Answer from the drawing. Dimensions are ordinates in mm from the lowest x, y and z of the part. Coordinates: 2 decimals unless noted, no trailing zeros. Write each loop counter-clockwise with the first axis right and the second up, starting at its lowest first coordinate (ties: lowest second). Pieces come first, ordered by that corner, then holes. Notation, with made-up numbers: (5, -7) -> (50, -7) arc R18 ccw to (50, 11) -> close; hole circle Ø4 at (60, 56). An arc over 180 degrees is marked (long way). Use CSV: the item, a comma, the result in double quotes.
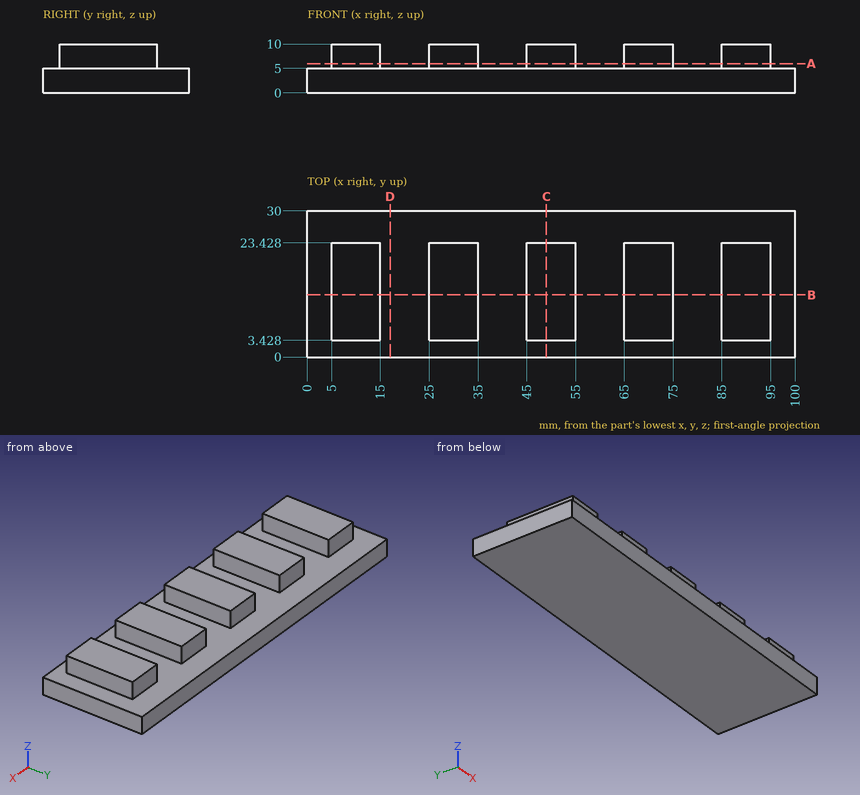
1. A cutting plane is placed at D-D (x = 17). Give the vertices of the cut face in (y, z), and give its area (3 significant figures).
Solutions:
outline,"(0, 0) -> (30, 0) -> (30, 5) -> (0, 5) -> close"
area,"150 mm^2"
2. A cutting plane is placed at B-B (y = 12.75). Give the vertices of the cut face in (x, z), and give its area (3 significant figures).
Solutions:
outline,"(0, 0) -> (100, 0) -> (100, 5) -> (95, 5) -> (95, 10) -> (85, 10) -> (85, 5) -> (75, 5) -> (75, 10) -> (65, 10) -> (65, 5) -> (55, 5) -> (55, 10) -> (45, 10) -> (45, 5) -> (35, 5) -> (35, 10) -> (25, 10) -> (25, 5) -> (15, 5) -> (15, 10) -> (5, 10) -> (5, 5) -> (0, 5) -> close"
area,"750 mm^2"
3. A cutting plane is placed at C-C (x = 49). Give the vertices of the cut face in (y, z).
Solutions:
outline,"(0, 0) -> (30, 0) -> (30, 5) -> (23.43, 5) -> (23.43, 10) -> (3.43, 10) -> (3.43, 5) -> (0, 5) -> close"
4. Each of these flat-tipped pins is pushed along its axis until it touches: pin 1 Ø5 at (x, y) = (77.5, 26) entering from +Z; pin 2 Ø4 at (y, z) = (7.5, 8) entering from +X; pin 3 Ø1.5 at (y, z) = (13, 7) entering from -X. Where does it stop, or does it pass through?
Solutions:
pin 1,"stops at z = 5"
pin 2,"stops at x = 95"
pin 3,"stops at x = 5"
5. A cutting plane is placed at A-A (z = 6). Give the vertices of the cut face in (x, y).
Solutions:
outline,"(5, 3.43) -> (15, 3.43) -> (15, 23.43) -> (5, 23.43) -> close; (25, 3.43) -> (35, 3.43) -> (35, 23.43) -> (25, 23.43) -> close; (45, 3.43) -> (55, 3.43) -> (55, 23.43) -> (45, 23.43) -> close; (65, 3.43) -> (75, 3.43) -> (75, 23.43) -> (65, 23.43) -> close; (85, 3.43) -> (95, 3.43) -> (95, 23.43) -> (85, 23.43) -> close"
6. Find the intervals of material crossed by line 1 along X through (y, z) = (19.25, 5.5); line 2 along Y through (x, z) = (71.5, 6.5); line 3 along Z through (x, y) = (16, 11.5), in increasing order.
Solutions:
line 1,"x = 5 to 15, 25 to 35, 45 to 55, 65 to 75, 85 to 95"
line 2,"y = 3.43 to 23.43"
line 3,"z = 0 to 5"
